```python
from build123d import *

# Parameters (mm, degrees)
EXTRUDE_1_DEPTH = 600


with BuildPart() as part:
    # Эскиз1 → Бобышка-Вытянуть1 (new body)
    with BuildSketch(Plane(origin=(0, 0, 0), x_dir=(1, 0, 0), z_dir=(0, 1, 0))):
        with BuildLine():
            Line((5, 0), (820, 0))
            Line((820, 0), (820, 18.800386004))
            Line((820, 18.800386004), (785.363179306, 18.800386004))
            Line((785.363179306, 18.800386004), (785.363179306, 45))
            Line((785.363179306, 45), (0, 45))
            Line((0, 45), (0, 5))
            ThreePointArc((0, 5), (-3.535533906, -3.535533906), (5, 0))
        make_face()
    extrude(amount=EXTRUDE_1_DEPTH)


solid = part.part
```
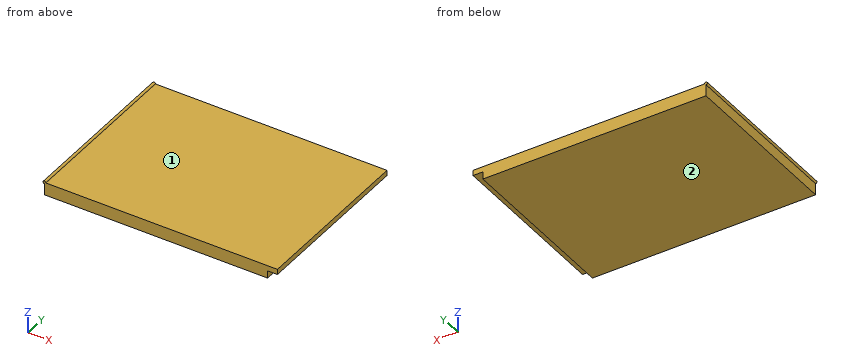
Verification items for the finished model (mm, model axes). Face numbers are marked on the shaded views. A direction names the side the tool comes from. Coordinates: 2 decimals unless noted, no trailing zeros. Order: outer loops, then holes, each group sorted by start corner. A loop starts at its lowest first (then second) coordinate and runs counter-clockwise, first axis right, second up. Notation, with made-up numbers: (44, -19) - (68, -19) arc R15 cw to (68, -10) - close; hole circle Ø5 at (76, 78). An arc over 180 degrees is marked (long way). Return JSON: item names as keys, results as strings.
(1) Section check B-B, the plane z = -32.5. Record the cut outline in (x, y), and give its area (3 significant figures).
Filled sheet:
{"outline": "(0, 0) - (785.36, 0) - (785.36, 600) - (0, 600) - close", "area": "471,000 mm^2"}
(2) Section check C-C, the plane x = 415. Record the cut outline in (y, z), and give its area (3 significant figures).
Filled sheet:
{"outline": "(0, -45) - (600, -45) - (600, 0) - (0, 0) - close", "area": "27,000 mm^2"}
(3) Go/stop test with flat-tipped pins: pin 1 (17.5 mm diameter, centred on x = 811, y = 369, fed in from -Z); pin 2 (12 mm diameter, centred on x = 168.5, y = 319.5, fed in from +Z); pin 3 (12 mm diameter, centred on y = 229, z = -33, fed in from -X). Record where each tip stops, or that it passes through.
Filled sheet:
{"pin 1": "stops at z = -18.8", "pin 2": "stops at z = 0", "pin 3": "stops at x = 0"}
(4) Thickness scan on line 1 along X through (y, z) = (192.5, -7); line 2 along Z through (x, y) = (597, 333); line 3 along X through (y, z) = (188, -41). Record the ranges inside material, lowest first.
Filled sheet:
{"line 1": "x = 0 to 820", "line 2": "z = -45 to 0", "line 3": "x = 0 to 785.36"}
(5) Access from +Z, -Z, +X, -X, +Y, -Y to the whole of each face (thin tool, end or side, straight path). Record for the marked faces 1 and 2.
Filled sheet:
{"face 1": "+Z, +X, +Y, -Y", "face 2": "-Z, +X, -X, +Y, -Y"}
(6) Section check A-A, the plane y = 167. Record the cut outline in (x, z).
Filled sheet:
{"outline": "(0, -45) - (785.36, -45) - (785.36, -18.8) - (820, -18.8) - (820, 0) - (5, 0) arc R5 ccw (long way) to (0, -5) - close"}
